from build123d import *

# Parameters (mm, degrees)
SKETCH1_W          = 40
SKETCH1_H          = 130
SKETCH1_R          = 6.35
SKETCH1_R_2        = 3.175
BASE_FLANGE1_DEPTH = 3.175
EDGE_FLANGE1_DEPTH = 40
EDGE_FLANGE2_DEPTH = 40
SKETCH20_R         = 3.175
CUT_EXTRUDE3_DEPTH = 3.175


# Sheet-metal steps are written as plain solids
with BuildPart() as part:
    # Sketch1 → Base-Flange1 (new body)
    with BuildSketch(Plane(origin=(0, 0, 0), x_dir=(0, 0, -1), z_dir=(1, 0, 0))):
        with Locations((20, -65)):
            Rectangle(SKETCH1_W, SKETCH1_H)
        with Locations((20, -20)):
            Circle(SKETCH1_R, mode=Mode.SUBTRACT)
        with Locations((20, -64.45)):
            Circle(SKETCH1_R_2, mode=Mode.SUBTRACT)
    extrude(amount=-BASE_FLANGE1_DEPTH)

    # Edge-Flange1 section (across the edge) → Edge-Flange1 (add)
    with BuildSketch(Plane(origin=(0, -130.268100475, 0), x_dir=(0.7660444431189817, 0.642787609686535, 0), z_dir=(0, 0, -1))):
        with BuildLine():
            Line((-3.175, 0.268100475), (-3.175, 25))
            Line((-3.175, 25), (0, 25))
            Line((0, 25), (0, 0.268100475))
            ThreePointArc((0, 0.268100475), (0.044422416, 0.016168437), (0.172331663, -0.205376879))
            Line((0.172331663, -0.205376879), (-2.259859444, -2.246227539))
            ThreePointArc((-2.259859444, -2.246227539), (-2.939101655, -1.069745518), (-3.175, 0.268100475))
        make_face()
    extrude(amount=EDGE_FLANGE1_DEPTH)

    # Edge-Flange2 section (across the edge) → Edge-Flange2 (add)
    with BuildSketch(Plane(origin=(13.809830798, -151.665439092, -40), x_dir=(-1, 0, 0), z_dir=(0, 0, 1))):
        with BuildLine():
            Line((-3.175, 0.268100475), (-3.175, 30))
            Line((-3.175, 30), (0, 30))
            Line((0, 30), (0, 0.268100475))
            ThreePointArc((0, 0.268100475), (0.044422416, 0.016168437), (0.172331663, -0.205376879))
            Line((0.172331663, -0.205376879), (-2.259859444, -2.246227539))
            ThreePointArc((-2.259859444, -2.246227539), (-2.939101655, -1.069745518), (-3.175, 0.268100475))
        make_face()
    extrude(amount=EDGE_FLANGE2_DEPTH)

    # Sketch20 → Cut-Extrude3 (cut)
    with BuildSketch(Plane(origin=(16.984830798, 0, 0), x_dir=(0, 0, -1), z_dir=(1, 0, 0))):
        with Locations(Location((20, -166.799489329, 0), (0, 0, 90))):
            Circle(SKETCH20_R)
    extrude(amount=-CUT_EXTRUDE3_DEPTH, mode=Mode.SUBTRACT)


solid = part.part
Read the model definition and answer for the solid it produces. Units are mm, in the model's axes. A direction names the side the tool comes from. Round coordinates to 2 decimals unless told otherwise and drop trailing zeros. Write each loop counter-clockwise with the first axis right and the second up, starting at its lowest first coordinate (ties: lowest second). Pieces come first, ordered by that corner, then holes.
1. Given pin 1 Ø20 at (y, z) = (-83, -28) entering from +X; pin 2 Ø10 at (y, z) = (-20, -20) entering from -X; pin 3 Ø2 at (x, z) = (0.5, -28.5) entering from +Y; pin 4 Ø1 at (x, z) = (4.5, -17.5) entering from -Y, each flat-ended and moving along its own axis, determine where each tip first touches the part or whether it passes through.
2. The part is cut by section A-A, the plane z = -20. State how many separate pieces and enclosed holes the cut face has, then the cut area to 3 significant figures.
3. Straight lines are drawn through the part: L1, parallel to Y at x = -2.4, z = -20 (3 decimals); L2, parallel to Y at x = -1.2, z = -20 (3 decimals); L3, parallel to Y at x = -1, z = -16.5. For each, find the intervals that lie inside material, in ascending order.
4. The part is cut by section D-D, the plane y = -20. Determine the outline of the cut face in (x, z) (3 decimals), then the cut area to 3 significant figures.
5. Determine the mould class of faces 1 (the face through (-2, 0, -20)), 2 (the face through (-1.565, -62.304, -17.66)), 3 (the face through (-1, -91, 0)) for opening direction Y: pulls with the +Y half, pulls with the -Y half, needs draft (parallel to the pull), parting line crosses it, or undercut.
6. The part is cut by section C-C, the plane z = -12. Determine the outline of the cut face in (x, y) (1 decimal).
7. Which of the six approach directions +Z, -Z, +X, -X, +Y, -Y give full straight-line access (tool end or side, diameter ignored) to faces 4 (the face through (13.81, -170.3, -20.3)), 5 (the face through (0, -64, -24)), 6 (the face through (16.985, -163, -20))?
8. The part is cut by section B-B, the plane y = -64.45. Determine the outline of the cut face in (x, z) (3 decimals), then the cut area to 3 significant figures.
Values:
1. pin 1: stops at x = 0
1. pin 2: passes through
1. pin 3: stops at y = 0
1. pin 4: stops at y = -141.17
2. separate pieces: 4
2. enclosed holes: 0
2. area: 515 mm2
3. L1: y = -132.337 to -67.625, -61.275 to -26.35, -13.65 to 0
3. L2: y = -133.777 to -67.625, -61.275 to -26.35, -13.65 to 0
3. L3: y = -134.02 to -25.3, -14.7 to 0
4. outline: (-3.175, -40) - (0, -40) - (0, -26.35) - (-3.175, -26.35) - close; (-3.175, -13.65) - (0, -13.65) - (0, 0) - (-3.175, 0) - close
4. area: 86.7 mm2
5. face 1: pulls with the +Y half
5. face 2: undercut
5. face 3: needs draft
6. outline: (-3.2, -130) arc R3.9 ccw to (-2.3, -132.5) - (13.6, -151.5) arc R0.7 cw to (13.8, -151.9) - (13.8, -181.7) - (17, -181.7) - (17, -151.9) arc R3.9 ccw to (16.1, -149.4) - (0.2, -130.5) arc R0.7 cw to (0, -130) - (0, 0) - (-3.2, 0) - close
7. face 4: +Z, -Z, -X, -Y
7. face 5: +Z, -Z, +X, +Y
7. face 6: +Z, -Z, +X, +Y, -Y
8. outline: (-3.175, -40) - (0, -40) - (0, -23.175) - (-3.175, -23.175) - close; (-3.175, -16.825) - (0, -16.825) - (0, 0) - (-3.175, 0) - close
8. area: 107 mm2
